```python
from build123d import *

# Parameters (mm, degrees)
ESQUISSE1_W        = 36.7
ESQUISSE1_H        = 26.5
BOSS_EXTRU_2_DEPTH = 1
ESQUISSE1_2_W      = 37.5
ESQUISSE1_2_H      = 27.3
ESQUISSE1_2_W_2    = 36.7
ESQUISSE1_2_H_2    = 26.5
EXTRU_MINCE1_DEPTH = 4


with BuildPart() as part:
    # Esquisse1 → Boss.-Extru.2 (new body)
    with BuildSketch(Plane.XY):
        Rectangle(ESQUISSE1_W, ESQUISSE1_H)
    extrude(amount=BOSS_EXTRU_2_DEPTH)

    # Esquisse1<2> → Extru.-Mince1 (add)
    with BuildSketch(Plane.XY):
        Rectangle(ESQUISSE1_2_W, ESQUISSE1_2_H)
        Rectangle(ESQUISSE1_2_W_2, ESQUISSE1_2_H_2, mode=Mode.SUBTRACT)
    extrude(amount=EXTRU_MINCE1_DEPTH)


solid = part.part
```
Source: CAD feature listing. Evaluate the final solid. Frame: model axes, mm. A direction names the side the tool comes from. Coordinates: 2 decimals unless noted, no trailing zeros. Order: outer loops, then holes, each group sorted by start corner. A loop starts at its lowest first (then second) coordinate and runs counter-clockwise, first axis right, second up. Notation, with made-up numbers: (62.5, 71.25) - (77.5, 71.25) arc R20 cw to (77.5, 106.25) - close; hole circle Ø10 at (-5, -1). An arc over 180 degrees is marked (long way). One line per item, written item: value.
1) Cut plane B-B on x = 9. Output: boundary loops of the cut face in (y, z), plus the area to 3 significant figures.
Computed values:
outline: (-13.65, 0) - (13.65, 0) - (13.65, 4) - (13.25, 4) - (13.25, 1) - (-13.25, 1) - (-13.25, 4) - (-13.65, 4) - close
area: 29.7 mm^2
2) Reachability of faces 4 (the face through (0, 0, 0)), 5 (the face through (0, 13.25, 2)) from +Z, -Z, +X, -X, +Y, -Y: full face, straight path, thin tool, end or side. Return the list, or none.
Computed values:
face 4: -Z, +X, -X, +Y, -Y
face 5: +Z
3) Cut plane C-C on y = 7. Output: boundary loops of the cut face in (x, z).
Computed values:
outline: (-18.75, 0) - (18.75, 0) - (18.75, 4) - (18.35, 4) - (18.35, 1) - (-18.35, 1) - (-18.35, 4) - (-18.75, 4) - close
4) Cut plane A-A on z = 3.6. Output: boundary loops of the cut face in (x, y), plus the area to 3 significant figures.
Computed values:
outline: (-18.75, -13.65) - (18.75, -13.65) - (18.75, 13.65) - (-18.75, 13.65) - close; hole (-18.35, -13.25) - (18.35, -13.25) - (18.35, 13.25) - (-18.35, 13.25) - close
area: 51.2 mm^2
5) Contact query for a flat-ended pin moving along its axis: pin 1 (2 mm diameter, centred on x = 10.5, y = -4.5, fed in from +Z). Output: stop coordinate, or through.
Computed values:
pin 1: stops at z = 1
6) Mould query, pull axis X, two halves, no side actions, for faces 1 (the face through (0, 0, 1)), 2 (the face through (0, -13.65, 2)), 3 (the face through (-18.75, 0, 2)). Classes: released by +X, released by -X, zero draft, split by the parting line, or undercut.
Computed values:
face 1: undercut
face 2: zero draft
face 3: released by -X
7) Ray query, line 1 (X direction, y = -12.25, z = 3.3); line 2 (Y direction, x = -7, z = 2.75); line 3 (Z direction, x = -1.5, y = -1.25). Return the intervals inside material, ascending. Write a range as [from, to].
Computed values:
line 1: x = [-18.75, -18.35], [18.35, 18.75]
line 2: y = [-13.65, -13.25], [13.25, 13.65]
line 3: z = [0, 1]
